Verification items for this drawing (mm, ordinates from the low corner). Round coordinates to 2 decimals unless told otherwise and drop trailing zeros. Loops run counter-clockwise (first coordinate to the right, second up) from the corner with the lowest first, then second, coordinate; pieces in that order, holes last. Notation, with made-up numbers: M 51,28 L 67,28 A19 cw 67,61 Z; hole C -14.75,5 d11. An arc over 180 degrees is marked long. Use one line per item in the form item = value. Start each with the question number.
1. Cross-section at D-D (z = 26.5). Record the boundary of the cut face in (x, y), then the cut area to 3 significant figures.
2. Draft check along X on the marked faces 1 and 2. Enter one of: pulls with the +X half, pulls with the -X half, needs draft (parallel to the pull), parting line crosses it, or undercut.
3. Cross-section at B-B (z = 3). Record the boundary of the cut face in (x, y).
4. Cross-section at A-A (y = 3). Record the boundary of the cut face in (x, z), then the cut area to 3 significant figures.
5. Go/stop test with flat-tipped pins: pin 1 (1.2 mm diameter, centred on x = 5.5, z = 34.5, fed in from -Y); pin 2 (21 mm diameter, centred on y = 35, z = 57.5, fed in from +X); pin 3 (12 mm diameter, centred on y = 45, z = 22.5, fed in from -X). Record where each tip stops, or that it passes through.
6. Cross-section at C-C (x = 4). Record the boundary of the cut face in (y, z), then the cut area to 3 significant figures.
7. Material ranges on line 1 (Y direction, x = 1.5, z = 87); line 2 (Z direction, x = 4.75, y = 73); line 3 (Y direction, x = 5.75, z = 87), recorded low to high.
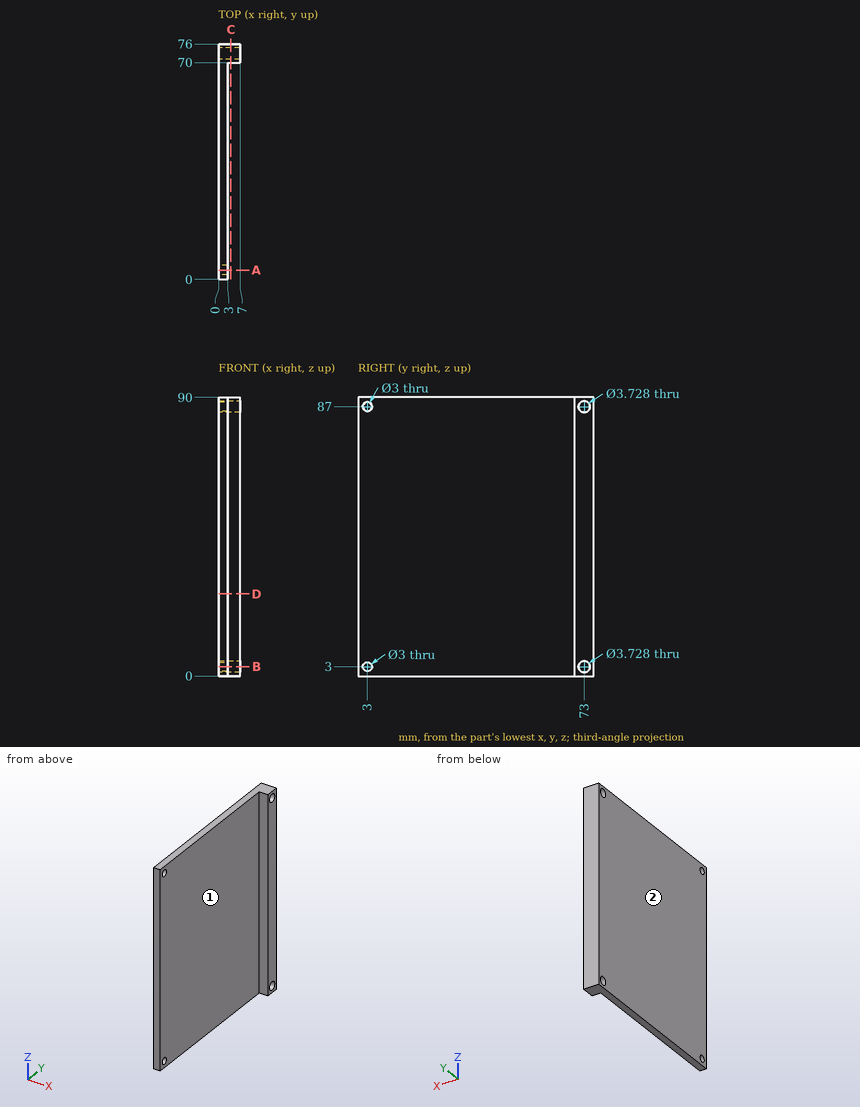
Reported:
q1.outline = M 0,0 L 3,0 L 3,70 L 7,70 L 7,76 L 0,76 Z
q1.area = 252 mm²
q2.face_1 = pulls with the +X half
q2.face_2 = pulls with the -X half
q3.outline = M 0,0 L 3,0 L 3,1.5 L 0,1.5 Z; M 0,4.5 L 3,4.5 L 3,70 L 7,70 L 7,71.14 L 0,71.14 Z; M 0,74.86 L 7,74.86 L 7,76 L 0,76 Z
q4.outline = M 0,0 L 3,0 L 3,1.5 L 0,1.5 Z; M 0,4.5 L 3,4.5 L 3,85.5 L 0,85.5 Z; M 0,88.5 L 3,88.5 L 3,90 L 0,90 Z
q4.area = 252 mm²
q5.pin_1 = 70
q5.pin_2 = 3
q5.pin_3 = 0
q6.outline = M 70,0 L 76,0 L 76,90 L 70,90 Z; hole C 73,3 d3.73; hole C 73,87 d3.73
q6.area = 518 mm²
q7.line_1 = 0 to 1.5, 4.5 to 71.14, 74.86 to 76
q7.line_2 = 0 to 1.14, 4.86 to 85.14, 88.86 to 90
q7.line_3 = 70 to 71.14, 74.86 to 76
